```python
from build123d import *

# Parameters (mm, degrees)
CROQUIS1_W              = 42
CROQUIS1_H              = 12
CROQUIS1_R              = 1.6
SALIENTE_EXTRUIR1_DEPTH = 2
CROQUIS2_W              = 12
CROQUIS2_H              = 12
SALIENTE_EXTRUIR2_DEPTH = 7
CROQUIS3_R              = 2
SALIENTE_EXTRUIR3_DEPTH = 6.5
CROQUIS4_R              = 4.5
SALIENTE_EXTRUIR4_DEPTH = 3
REDONDEO1_R             = 1


with BuildPart() as part:
    # Croquis1 → Saliente-Extruir1 (new body)
    with BuildSketch(Plane(origin=(0, 0, 0), x_dir=(1, 0, 0), z_dir=(0, 1, 0))):
        Rectangle(CROQUIS1_W, CROQUIS1_H)
        with Locations(Location((-15, 0, 0), (0, 0, 270))):
            Circle(CROQUIS1_R, mode=Mode.SUBTRACT)
        with Locations(Location((15, 0, 0), (0, 0, 270))):
            Circle(CROQUIS1_R, mode=Mode.SUBTRACT)
    extrude(amount=SALIENTE_EXTRUIR1_DEPTH)

    # Croquis2 → Saliente-Extruir2 (add)
    with BuildSketch(Plane(origin=(0, 2, 0), x_dir=(1, 0, 0), z_dir=(0, 1, 0))):
        Rectangle(CROQUIS2_W, CROQUIS2_H)
    extrude(amount=SALIENTE_EXTRUIR2_DEPTH)

    # Croquis3 → Saliente-Extruir3 (add)
    with BuildSketch(Plane(origin=(0, 9, 0), x_dir=(1, 0, 0), z_dir=(0, 1, 0))):
        with Locations(Location((0, 0, 0), (0, 0, 90))):
            Circle(CROQUIS3_R)
    extrude(amount=SALIENTE_EXTRUIR3_DEPTH)

    # Croquis4 → Saliente-Extruir4 (add)
    with BuildSketch(Plane(origin=(0, 15.5, 0), x_dir=(1, 0, 0), z_dir=(0, 1, 0))):
        with Locations(Location((0, 0, 0), (0, 0, 270))):
            Circle(CROQUIS4_R)
    extrude(amount=SALIENTE_EXTRUIR4_DEPTH)

    # Redondeo1
    redondeo1_edges = [part.edges().sort_by_distance(p)[0] for p in [
        (0, 9, 2),
    ]]
    fillet(redondeo1_edges, radius=REDONDEO1_R)


solid = part.part
```
Design review of the part built by this model. Coordinates are the model's own, in mm. A direction names the side the tool comes from. Give positions to 0.01 mm unless a question says otherwise; leave off trailing zeros. Order: outer loops, then holes, each group sorted by start corner. A loop starts at its lowest first (then second) coordinate and runs counter-clockwise, first axis right, second up. Notation, with made-up numbers: (0.25, 89.25) -> (57.25, 89.25) arc R32 ccw to (57.25, 121.25) -> close; hole circle Ø9 at (85, 22.25). An arc over 180 degrees is marked (long way). Write item = value, one per line. Start each with the question number.
(1) Mouldability with a two-part tool opening along Y and no side actions: class faces 1 (the face through (-3, 9, -1)), 2 (the face through (0, 3, 6)), 3 (the face through (0, 0, 0)) as +Y half, -Y half, draft (parallel to the pull), parting line (faces both ways), or undercut.
(2) To check wall thickness, follow line 1 along X through (y, z) = (0.8, 0); line 2 along Y through (x, z) = (-3.5, 0.5); line 3 along Y through (x, z) = (-18, 4.25). State the ranges of each line that lie inside material, in increasing order.
(3) We need section A-A on z = 0. Write out the cut boundary in (x, y), plus the area to 3 significant figures.
(4) For faces 4 (the face through (2, 13, 0)), 5 (the face through (13, 2, 0)), 6 (the face through (-6, 5, 0)), list the 3-axis set-ups (+Z, -Z, +X, -X, +Y, -Y) from which the entire face can be reached by the end or side of a thin tool; tool diameter is ignored.
(5) We need section B-B on x = -15. Write out the cut boundary in (y, z), plus the area to 3 significant figures.
(6) For pin 1 (1.5 mm diameter, centred on y = 16, z = -4.5, fed in from -X); pin 2 (6 mm diameter, centred on x = -10, z = -1, fed in from +Y); pin 3 (2.5 mm diameter, centred on x = 1, z = -1, fed in from -Y); pin 4 (5 mm diameter, centred on y = 10.5, z = -2.5, fed in from -X), all flat-tipped, find the tip position at first contact; note any pin that passes through.
(7) We need section C-C on x = 0. Write out the cut boundary in (y, z).
(8) We need section D-D on y = 6.5. Write out the cut boundary in (x, z).
Numbers:
q1.face_1 = undercut
q1.face_2 = draft
q1.face_3 = -Y half
q2.line_1 = -21 to -16.6, -13.4 to 13.4, 16.6 to 21
q2.line_2 = 0 to 9, 15.5 to 18.5
q2.line_3 = 0 to 2
q3.outline = (-21, 0) -> (-16.6, 0) -> (-16.6, 2) -> (-21, 2) -> close; (-13.4, 0) -> (13.4, 0) -> (13.4, 2) -> (6, 2) -> (6, 9) -> (3, 9) arc R1 cw to (2, 10) -> (2, 15.5) -> (4.5, 15.5) -> (4.5, 18.5) -> (-4.5, 18.5) -> (-4.5, 15.5) -> (-2, 15.5) -> (-2, 10) arc R1 cw to (-3, 9) -> (-6, 9) -> (-6, 2) -> (-13.4, 2) -> close; (16.6, 0) -> (21, 0) -> (21, 2) -> (16.6, 2) -> close
q3.area = 209 mm^2
q4.face_4 = none
q4.face_5 = +Z, -Z, +X, +Y
q4.face_6 = +Z, -Z, -X, +Y
q5.outline = (0, -6) -> (2, -6) -> (2, -1.6) -> (0, -1.6) -> close; (0, 1.6) -> (2, 1.6) -> (2, 6) -> (0, 6) -> close
q5.area = 17.6 mm^2
q6.pin_1 = -2.49
q6.pin_2 = 2
q6.pin_3 = 0
q6.pin_4 = -6
q7.outline = (0, -6) -> (9, -6) -> (9, -3) arc R1 cw to (10, -2) -> (15.5, -2) -> (15.5, -4.5) -> (18.5, -4.5) -> (18.5, 4.5) -> (15.5, 4.5) -> (15.5, 2) -> (10, 2) arc R1 cw to (9, 3) -> (9, 6) -> (0, 6) -> close
q8.outline = (-6, -6) -> (6, -6) -> (6, 6) -> (-6, 6) -> close
